```python
from build123d import *

# Parameters (mm, degrees)
BOSS_EXTRUDE1_DEPTH = 4
BOSS_EXTRUDE1_DRAFT = 1
SHELL1_T            = -0.5
SKETCH2_R           = 2
BOSS_EXTRUDE2_DEPTH = 5.5
BOSS_EXTRUDE2_TAPER = 1.5
CIRPATTERN1_COUNT   = 4


with BuildPart() as part:
    # Sketch1 → Boss-Extrude1 (with draft: the straight prism first)
    with BuildSketch(Plane(origin=(0, 0, 0), x_dir=(1, 0, 0), z_dir=(0, 1, 0))):
        with BuildLine():
            Line((-7.5, -6.375), (7.5, -6.375))
            ThreePointArc((7.5, -6.375), (8.207106781, -6.082106781), (8.5, -5.375))
            Line((8.5, -5.375), (8.5, 5.375))
            ThreePointArc((8.5, 5.375), (8.207106781, 6.082106781), (7.5, 6.375))
            Line((7.5, 6.375), (-7.5, 6.375))
            ThreePointArc((-7.5, 6.375), (-8.207106781, 6.082106781), (-8.5, 5.375))
            Line((-8.5, 5.375), (-8.5, -5.375))
            ThreePointArc((-8.5, -5.375), (-8.207106781, -6.082106781), (-7.5, -6.375))
        make_face()
    extrude(amount=-BOSS_EXTRUDE1_DEPTH)
    # Boss-Extrude1: the draft: its side faces are tilted about the plane it starts from
    boss_extrude1_sides = [part.faces().sort_by_distance(p)[0] for p in [
        (0, -2, 6.375),
        (8.207106781, -2, 6.082106781),
        (8.5, -2, 0),
        (8.207106781, -2, -6.082106781),
        (0, -2, -6.375),
        (-8.207106781, -2, -6.082106781),
        (-8.5, -2, 0),
        (-8.207106781, -2, 6.082106781),
    ]]
    draft(boss_extrude1_sides, Plane(origin=(0, 0, 0), x_dir=(1, 0, 0), z_dir=(0, 1, 0)), BOSS_EXTRUDE1_DRAFT)

    # Shell1
    shell1_openings = [part.faces().sort_by_distance(p)[0] for p in [
        (0, -4, 0),
    ]]
    offset(amount=SHELL1_T, openings=shell1_openings, kind=Kind.INTERSECTION)

    # Sketch2 → Boss-Extrude2 (add)
    with BuildSketch(Plane.XZ.offset(0.5)):
        Circle(SKETCH2_R)
    extrude(amount=BOSS_EXTRUDE2_DEPTH, taper=BOSS_EXTRUDE2_TAPER)

    # Rib1: read off the stored shape, not the designer's step
    # Rib1: loft between two sections, ruled curve by curve
    rib1_from = [
        Edge.make_line((1.982020214, -0.5, 0.267574046), (3, -0.5, 0.25)),
        Edge.make_line((1.982020214, -0.5, -0.267574046), (3, -0.5, -0.25)),
        Edge.make_line((3, -0.5, -0.25), (3, -0.5, 0.25)),
        Edge.make_line((1.982020214, -0.5, -0.267574046), (1.982020214, -0.5, 0.267574046)),
    ]
    rib1_to = [
        Edge.make_line((1.877466543, -4.5, 0.259067318), (2.402692557, -4.5, 0.25)),
        Edge.make_line((1.877466543, -4.5, -0.259067318), (2.402692557, -4.5, -0.25)),
        Edge.make_line((2.402692557, -4.5, -0.25), (2.402692557, -4.5, 0.25)),
        Edge.make_line((1.877466543, -4.5, -0.259067318), (1.877466543, -4.5, 0.259067318)),
    ]
    rib1 = Solid(Shell([*[Face.make_surface_from_curves(rib1_from[k], rib1_to[k]) for k in range(4)], Face(Wire(rib1_from)), Face(Wire(rib1_to))]))
    add(rib1)

    # CirPattern1: Rib1 ×4 about axis
    cirpattern1_axis = Axis((0, 0, 0), (0, 1, 0))
    for i in range(1, CIRPATTERN1_COUNT):
        add(rib1.rotate(cirpattern1_axis, i * 360 / CIRPATTERN1_COUNT))


solid = part.part
```
Geometry check sheet. Reference: the model listing, model coordinates, mm. A direction names the side the tool comes from. Coordinates: 2 decimals unless noted, no trailing zeros. Order: outer loops, then holes, each group sorted by start corner. A loop starts at its lowest first (then second) coordinate and runs counter-clockwise, first axis right, second up. Notation, with made-up numbers: (28.25, 24.5) - (64.25, 24.5) arc R21 ccw to (64.25, 62.5) - close; hole circle Ø9 at (-39.5, -2). An arc over 180 degrees is marked (long way). Answer in a Markdown table with one row per item. Add a question column.
1. Material ranges on L1, parallel to X at y = -3, z = -1.25; L2, parallel to X at y = -2, z = -0.5; L3, parallel to Z at x = -1.25, y = -2.25, recorded low to high. Write a range as [from, to].
2. Section check B-B (z = -4.75). Enter the section's corners in (x, y), plus the area to 3 significant figures.
3. Access from +Z, -Z, +X, -X, +Y, -Y to the whole of each face (thin tool, end or side, straight path). Record for faces 1 (the face through (-8.223, -1.972, -6.114)), 2 (the face through (0.89, -3.29, -1.71)), 3 (the face through (8.223, -1.972, 6.114)).
4. Gauge pin test, flat ends, axial feed: pin 1 Ø1.5 at (x, y) = (4, -1.5) entering from +Z; pin 2 Ø1 at (x, y) = (-0.5, -2) entering from -Z. Record the tip position at first contact, or that the pin passes through.
5. Section check A-A (x = 3.5). Enter the section's corners in (y, z) (3 decimals), plus the area to 3 significant figures.
6. Draft check along X on faces 4 (the face through (0, -4, -6.2)), 5 (the face through (-2, -0.5, 1)), 6 (the face through (-8.24, -1.97, 6.1)). Enter one of: +X half, -X half, draft (parallel to the pull), parting line (faces both ways), or undercut.
7. Section check C-C (y = -1). Give the number of separate pieces and of enclosed holes in the cut face, plus the area to 3 significant figures.
Data:
| question | item | result |
|---|---|---|
| 1 | L1 | x = [-8.55, -8.05], [-1.48, 1.48], [8.05, 8.55] |
| 1 | L2 | x = [-8.53, -8.03], [-1.9, 1.9], [8.03, 8.53] |
| 1 | L3 | z = [-6.41, -5.91], [-1.5, 1.5], [5.91, 6.41] |
| 2 | outline | (-8.57, -4) - (-8.07, -4) - (-8.01, -0.5) - (8.01, -0.5) - (8.07, -4) - (8.57, -4) - (8.5, 0) - (-8.5, 0) - close |
| 2 | area | 12.0 mm² |
| 3 | face 1 | -Z, -X, +Y |
| 3 | face 2 | -Y |
| 3 | face 3 | +Z, +X, +Y |
| 4 | pin 1 | stops at z = 6.41 |
| 4 | pin 2 | stops at z = -6.42 |
| 5 | outline | (-4, -6.445) - (0, -6.375) - (0, 6.375) - (-4, 6.445) - (-4, 5.945) - (-0.5, 5.884) - (-0.5, -5.884) - (-4, -5.945) - close |
| 5 | area | 9.88 mm² |
| 6 | face 4 | draft |
| 6 | face 5 | undercut |
| 6 | face 6 | -X half |
| 7 | separate pieces | 2 |
| 7 | enclosed holes | 1 |
| 7 | area | 42.5 mm² |
